The listing builds one solid part. Answer for the finished solid, in the listing's coordinates (mm). Face numbers are marked on the shaded views. A direction names the side the tool comes from. Coordinates: 2 decimals unless noted, no trailing zeros. Write each loop counter-clockwise with the first axis right and the second up, starting at its lowest first coordinate (ties: lowest second). Pieces come first, ordered by that corner, then holes.
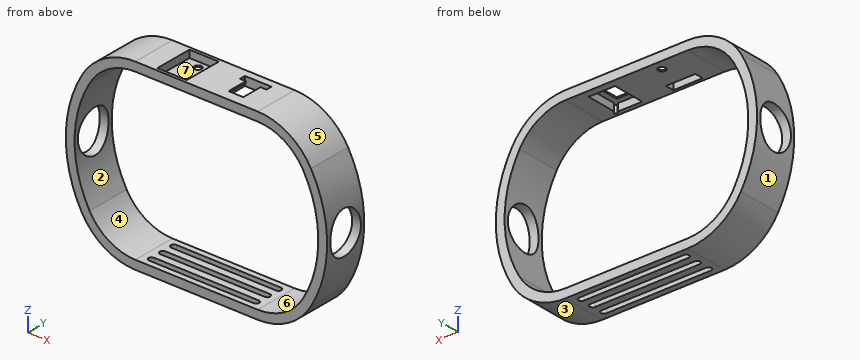
```python
from build123d import *

# Parameters (mm, degrees)
SKETCH_1_W           = 89
SKETCH_1_H           = 62
EXTRUDE_1_DEPTH      = 15
CUT_EXTRUDE_START    = -15.000001
SKETCH_2_W           = 114.345269922
SKETCH_2_H           = 82.741202996
CUT_EXTRUDE_2_DEPTH  = 15.000002
CUT_EXTRUDE_3_REACH  = 70.225
CUT_EXTRUDE_6_REACH  = 84.425
SKETCH_4_W           = 9
SKETCH_4_H           = 11
FILLET_1_R           = 0.5
CUT_EXTRUDE_7_REACH  = 82.193
EXTRUDE_2_DEPTH      = 0.5
SKETCH_11_W          = 10
SKETCH_11_H          = 13
CUT_EXTRUDE_10_DEPTH = 2.5
SKETCH_12_R          = 1.25
SKETCH_12_W          = 10
SKETCH_12_H          = 3
CUT_EXTRUDE_11_DEPTH = 2.5
CUT_EXTRUDE_12_REACH = 84.425
CUT_EXTRUDE_START_2  = -52.200000102
CUT_EXTRUDE_13_DEPTH = 88.999999964


with BuildPart() as part:
    # 草图1 → 凸台-拉伸1 (new body)
    with BuildSketch(Plane(origin=(0, 0, 0), x_dir=(1, 0, 0), z_dir=(0, 1, 0))):
        with Locations((-7.7, -10.288888889)):
            Rectangle(SKETCH_1_W, SKETCH_1_H)
    extrude(amount=EXTRUDE_1_DEPTH)

    # 草图2 → 切除-拉伸2 (cut)
    with BuildSketch(Plane(origin=(0, 15, 0), x_dir=(1, 0, 0), z_dir=(0, 1, 0)).offset(CUT_EXTRUDE_START)):
        with Locations((-11.341983823, -7.488413354)):
            Rectangle(SKETCH_2_W, SKETCH_2_H)
        with BuildLine():
            Line((-28.520508076, 20.711111111), (13.120508076, 20.711111111))
            ThreePointArc((13.120508076, 20.711111111), (23.620508076, 17.897644591), (31.307041555, 10.211111111))
            ThreePointArc((31.307041555, 10.211111111), (36.8, -10.288888889), (31.307041555, -30.788888889))
            ThreePointArc((31.307041555, -30.788888889), (23.620508076, -38.475422368), (13.120508076, -41.288888889))
            Line((13.120508076, -41.288888889), (-28.520508076, -41.288888889))
            ThreePointArc((-28.520508076, -41.288888889), (-39.020508076, -38.475422368), (-46.707041555, -30.788888889))
            ThreePointArc((-46.707041555, -30.788888889), (-52.2, -10.288888889), (-46.707041555, 10.211111111))
            ThreePointArc((-46.707041555, 10.211111111), (-39.020508076, 17.897644591), (-28.520508076, 20.711111111))
        make_face(mode=Mode.SUBTRACT)
    extrude(amount=CUT_EXTRUDE_2_DEPTH, mode=Mode.SUBTRACT)

    # 草图3 → 切除-拉伸3 (cut, up to next)
    with BuildSketch(Plane(origin=(0, 15, 0), x_dir=(1, 0, 0), z_dir=(0, 1, 0)), mode=Mode.PRIVATE) as cut_extrude_3_sk1:
        with BuildLine():
            Line((-28.520508076, -38.288888889), (13.120508076, -38.288888889))
            ThreePointArc((13.120508076, -38.288888889), (22.120508076, -35.877346157), (28.708965344, -29.288888889))
            ThreePointArc((28.708965344, -29.288888889), (33.8, -10.288888889), (28.708965344, 8.711111111))
            ThreePointArc((28.708965344, 8.711111111), (22.120508076, 15.299568379), (13.120508076, 17.711111111))
            Line((13.120508076, 17.711111111), (-28.520508076, 17.711111111))
            ThreePointArc((-28.520508076, 17.711111111), (-37.520508076, 15.299568379), (-44.108965344, 8.711111111))
            ThreePointArc((-44.108965344, 8.711111111), (-49.2, -10.288888889), (-44.108965344, -29.288888889))
            ThreePointArc((-44.108965344, -29.288888889), (-37.520508076, -35.877346157), (-28.520508076, -38.288888889))
        make_face()
    cut_extrude_3_tool1 = extrude(cut_extrude_3_sk1.sketch, amount=-CUT_EXTRUDE_3_REACH, mode=Mode.PRIVATE) & part.part
    add(cut_extrude_3_tool1.solids().sort_by_distance((-7.7, 15, 10.288889))[0], mode=Mode.SUBTRACT)

    # 草图4 → 切除-拉伸6 (cut, up to next)
    with BuildSketch(Plane.XY.offset(41.288888889), mode=Mode.PRIVATE) as cut_extrude_6_sk1:
        with Locations((2.8, 7)):
            Rectangle(SKETCH_4_W, SKETCH_4_H)
    cut_extrude_6_tool1 = extrude(cut_extrude_6_sk1.sketch, amount=-CUT_EXTRUDE_6_REACH, mode=Mode.PRIVATE) & part.part
    add(cut_extrude_6_tool1.solids().sort_by_distance((2.8, 7, 41.288889))[0], mode=Mode.SUBTRACT)

    # 圆角1
    fillet_1_edges = [part.edges().sort_by_distance(p)[0] for p in [
        (7.3, 1.5, 39.788888889),
    ]]
    fillet(fillet_1_edges, radius=FILLET_1_R)

    # 草图7 → 切除-拉伸7 (cut, up to next)
    with BuildSketch(Plane(origin=(0, 0, 38.288888889), x_dir=(-1, 0, 0), z_dir=(0, 0, -1)), mode=Mode.PRIVATE) as cut_extrude_7_sk1:
        Polygon((-7.3, 2.207106781), (-6.592893219, 1.5), (-7.3, 0.792893219), (-8.007106781, 1.5), align=None)
    cut_extrude_7_tool1 = extrude(cut_extrude_7_sk1.sketch, amount=-CUT_EXTRUDE_7_REACH, mode=Mode.PRIVATE) & part.part
    add(cut_extrude_7_tool1.solids().sort_by_distance((7.3, 1.5, 38.288889))[0], mode=Mode.SUBTRACT)

    # 草图8 → 凸台-拉伸2 (add)
    with BuildSketch(Plane.XY.offset(41.288888889)):
        Polygon((-1.7, 1.5), (-1.7, 0), (10.425334972, 0), (10.425334972, 10.5), (7.3, 10.5), (5.3, 10.5), (5.3, 3.5), (0.3, 3.5), (0.3, 10.5), (-1.7, 10.5), align=None)
    extrude(amount=-EXTRUDE_2_DEPTH)

    # 草图11 → 切除-拉伸10 (cut)
    with BuildSketch(Plane.XY.offset(41.288888889)):
        with Locations((-16.870478922, 7.5)):
            Rectangle(SKETCH_11_W, SKETCH_11_H)
    extrude(amount=-CUT_EXTRUDE_10_DEPTH, mode=Mode.SUBTRACT)

    # 草图12 → 切除-拉伸11 (cut)
    with BuildSketch(Plane.XY.offset(38.788888889)):
        with Locations((-16.870478922, 11.5)):
            Circle(SKETCH_12_R)
        with Locations((-16.870478922, 2.5)):
            Rectangle(SKETCH_12_W, SKETCH_12_H)
    extrude(amount=-CUT_EXTRUDE_11_DEPTH, mode=Mode.SUBTRACT)

    # 草图13 → 切除-拉伸12 (cut, up to next)
    with BuildSketch(Plane(origin=(0, 0, -20.711111111), x_dir=(-1, 0, 0), z_dir=(0, 0, -1)), mode=Mode.PRIVATE) as cut_extrude_12_sk1:
        with BuildLine():
            Line((-10.120508076, 13), (25.520508076, 13))
            ThreePointArc((25.520508076, 13), (26.520508076, 12), (25.520508076, 11))
            Line((25.520508076, 11), (-10.120508076, 11))
            ThreePointArc((-10.120508076, 11), (-11.120508076, 12), (-10.120508076, 13))
        make_face()
    cut_extrude_12_tool1 = extrude(cut_extrude_12_sk1.sketch, amount=-CUT_EXTRUDE_12_REACH, mode=Mode.PRIVATE) & part.part
    # 草图13 → 切除-拉伸12 (cut, up to next)
    with BuildSketch(Plane(origin=(0, 0, -20.711111111), x_dir=(-1, 0, 0), z_dir=(0, 0, -1)), mode=Mode.PRIVATE) as cut_extrude_12_sk2:
        with BuildLine():
            Line((-10.120508076, 6.5), (25.520508076, 6.5))
            ThreePointArc((25.520508076, 6.5), (26.520508076, 7.5), (25.520508076, 8.5))
            Line((25.520508076, 8.5), (-10.120508076, 8.5))
            ThreePointArc((-10.120508076, 8.5), (-11.120508076, 7.5), (-10.120508076, 6.5))
        make_face()
    cut_extrude_12_tool2 = extrude(cut_extrude_12_sk2.sketch, amount=-CUT_EXTRUDE_12_REACH, mode=Mode.PRIVATE) & part.part
    # 草图13 → 切除-拉伸12 (cut, up to next)
    with BuildSketch(Plane(origin=(0, 0, -20.711111111), x_dir=(-1, 0, 0), z_dir=(0, 0, -1)), mode=Mode.PRIVATE) as cut_extrude_12_sk3:
        with BuildLine():
            Line((-10.120508076, 2), (25.520508076, 2))
            ThreePointArc((25.520508076, 2), (26.520508076, 3), (25.520508076, 4))
            Line((25.520508076, 4), (-10.120508076, 4))
            ThreePointArc((-10.120508076, 4), (-11.120508076, 3), (-10.120508076, 2))
        make_face()
    cut_extrude_12_tool3 = extrude(cut_extrude_12_sk3.sketch, amount=-CUT_EXTRUDE_12_REACH, mode=Mode.PRIVATE) & part.part
    add(cut_extrude_12_tool1.solids().sort_by_distance((-7.7, 12, -20.711111))[0], mode=Mode.SUBTRACT)
    add(cut_extrude_12_tool2.solids().sort_by_distance((-7.7, 7.5, -20.711111))[0], mode=Mode.SUBTRACT)
    add(cut_extrude_12_tool3.solids().sort_by_distance((-7.7, 3, -20.711111))[0], mode=Mode.SUBTRACT)

    # 切除-拉伸13: read off the stored shape, not the designer's step
    # 切除-拉伸13 outline → 切除-拉伸13 (cut)
    with BuildSketch(Plane(origin=(0, 0, 0), x_dir=(0, 0, -1), z_dir=(1, 0, 0)).offset(CUT_EXTRUDE_START_2)):
        with BuildLine():
            add(Edge.make_bspline(
                [(-17.488888889, 7.5), (-17.488888889, 6.618712307), (-17.038806778, 4.85613692), (-15.30252013, 2.82180753), (-12.943624098, 1.578601929), (-10.288888889, 1.160699036), (-7.634153679, 1.578601929), (-5.275257648, 2.82180753), (-3.538970999, 4.85613692), (-2.863847834, 7.5), (-3.538970999, 10.14386308), (-5.275257648, 12.17819247), (-7.634153679, 13.421398071), (-10.288888889, 13.839300964), (-12.943624098, 13.421398071), (-15.30252013, 12.17819247), (-17.038806778, 10.14386308), (-17.488888889, 8.381287693), (-17.488888889, 7.5)],
                knots=[0, 0, 0, 0, 0.392699082, 0.785398163, 1.178097245, 1.570796327, 1.963495408, 2.35619449, 2.748893572, 3.141592654, 3.534291735, 3.926990817, 4.319689899, 4.71238898, 5.105088062, 5.497787144, 5.890486225, 6.283185307, 6.283185307, 6.283185307, 6.283185307], degree=3))
        make_face()
    extrude(amount=CUT_EXTRUDE_13_DEPTH, mode=Mode.SUBTRACT)


solid = part.part
```
(1) Section A-A, the plane x = -23 is taken. Write down the section's boundary in (y, z), plus the area to 3 significant figures.
(2) For a pull along X with two mould halves and no side action, classify the marked faces 1, 2, 3 and 4 as pulls with the +X half, pulls with the -X half, needs draft (parallel to the pull), parting line crosses it, or undercut.
(3) Each of these flat-tipped pins is pushed along its axis until it touches: pin 1 (3.5 mm diameter, centred on x = -5.5, z = -18.5, fed in from -Y); pin 2 (0.9 mm diameter, centred on y = 6, z = 39, fed in from +X); pin 3 (6 mm diameter, centred on y = 12, z = 3, fed in from +X); pin 4 (5 mm diameter, centred on x = -18.5, y = 5, fed in from +Z). Where does it stop, or does it pass through?
(4) Section B-B, the plane z = 23 is taken. Write down the section's boundary in (x, y).
(5) Which of the six approach directions +Z, -Z, +X, -X, +Y, -Y give full straight-line access (tool end or side, diameter ignored) to the marked faces 5, 6 and 7?
(6) Section C-C, the plane x = 26 is taken. Write down the section's boundary in (y, z), plus the area to 3 significant figures.
(7) Section D-D, the plane y = 7.5 is taken. State how many separate pieces and enclosed holes the cut face has, plus the area to 3 significant figures.
(8) Find the intervals of material crossed by probe 1 along Z at (x, y) = (-46.5, 1); probe 2 along Z at (x, y) = (2, 5.25); probe 3 along Z at (x, y) = (-24.5, 2.5), in increasing order.
Solution:
1. outline: (0, -20.71) - (2, -20.71) - (2, -17.71) - (0, -17.71) - close; (0, 38.29) - (15, 38.29) - (15, 41.29) - (0, 41.29) - close; (4, -20.71) - (6.5, -20.71) - (6.5, -17.71) - (4, -17.71) - close; (8.5, -20.71) - (11, -20.71) - (11, -17.71) - (8.5, -17.71) - close; (13, -20.71) - (15, -20.71) - (15, -17.71) - (13, -17.71) - close
1. area: 72.0 mm2
2. face 1: pulls with the -X half
2. face 2: undercut
2. face 3: pulls with the +X half
2. face 4: undercut
3. pin 1: stops at y = 0
3. pin 2: stops at x = 23.49
3. pin 3: stops at x = 36.57
3. pin 4: stops at z = 38.79
4. outline: (-50.18, 0) - (-47.01, 0) - (-47.01, 15) - (-50.18, 15) - close; (31.61, 0) - (34.78, 0) - (34.78, 15) - (31.61, 15) - close
5. face 5: +Z, +X, +Y, -Y
5. face 6: +Y, -Y
5. face 7: +Z
6. outline: (0, -16.3) - (15, -16.3) - (15, -12.29) - (0, -12.29) - close; (0, 32.86) - (15, 32.86) - (15, 36.88) - (0, 36.88) - close
6. area: 120 mm2
7. separate pieces: 4
7. enclosed holes: 0
7. area: 493 mm2
8. probe 1: z = -10.56 to -3.78, 24.36 to 31.14
8. probe 2: z = -20.71 to -17.71
8. probe 3: z = 38.29 to 41.29
